CAD build for the part. Positions are in the model's coordinates, mm. A direction names the side the tool comes from. Round coordinates to 2 decimals unless told otherwise and drop trailing zeros. Loops run counter-clockwise (first coordinate to the right, second up) from the corner with the lowest first, then second, coordinate; pieces in that order, holes last.
Autodesk Inventor part; units mm, degrees
ref_plane "Work Plane1" through (0, 9, -50) normal (0, 1, 0) x (-1, 0, 0)
ref_plane "Work Plane2" through (15.25, 0, 0) normal (1, 0, 0) x (0, 1, 0)
ref_plane "YZ Plane" through (0, 0, 0) normal (1, 0, 0) x (0, 1, 0)
sketch "Sketch1" plane through (0, 0, 0) normal (0, 0, 1) x (1, 0, 0)
  circle A0 centre (0, 0) radius 15.25
  dimension "d0" = 30.5
extrude "Extrusion1" add sketch "Sketch1" along normal blind 50
fillet "Fillet1" radius 2 1 edges at (-15.25, 0, 50)
fillet "Fillet2" radius 2 1 edges at (-15.25, 0, 0)
sketch "Sketch2" plane through (0, 0, 50) normal (0, 0, 1) x (1, 0, 0)
  circle A0 centre (0, 0) radius 9
  dimension "d5" = 18
extrude "Extrusion2" add sketch "Sketch2" along normal blind 184
sketch "Sketch3" plane through (0, 0, 0) normal (0, 0, -1) x (-1, 0, 0)
  circle A0 centre (0, 0) radius 9
extrude "Extrusion3" add sketch "Sketch3" along normal blind 50
sketch "Sketch4" plane through (0, 0, -50) normal (0, 0, -1) x (-1, 0, 0)
  circle A0 centre (0, 0) radius 3
  dimension "d10" = 6
extrude "Extrusion4" cut sketch "Sketch4" against normal blind 13
sketch "Sketch5" plane through (0, 0, -50) normal (0, 0, -1) x (-1, 0, 0)
  circle A0 centre (0, 0) radius 9
  point P0 (0, 9)
ref_plane "Work Plane1" through (0, 9, -50) normal (0, 1, 0) x (-1, 0, 0)
sketch "Sketch6" plane through (0, 9, -50) normal (0, 1, 0) x (-1, 0, 0)
  line L0 (-9, 0) -> (9, 0)
  point P0 (0, 50)
  point P1 (0, 5)
  dimension "d13" = 5
hole "Hole1" at (0, 9, -45) direction (0, -1, 0) diameter 3.242 depth 9 tip angle 118
sketch "Sketch7" plane through (0, 0, 0) normal (0, 0, -1) x (-1, 0, 0)
  circle A0 centre (0, 0) radius 15.25
  point P0 (-15.25, 0)
ref_plane "Work Plane2" through (15.25, 0, 0) normal (1, 0, 0) x (0, 1, 0)
sketch "Sketch8" plane through (15.25, 0, 0) normal (1, 0, 0) x (0, 1, 0)
  point P0 (0, 0)
  point P1 (0, 25)
  dimension "d21" = 25
hole "Hole2" at (15.25, 0, 25) direction (-1, 0, 0) diameter 3.242 end through all
sketch "Sketch9" plane through (0, 0, 234) normal (0, 0, 1) x (1, 0, 0)
  circle A0 centre (0, 0) radius 9
  line L0 (2.5, 8.9) -> (2.5, 6.5)
  line L1 (2.5, 6.5) -> (-2.5, 6.5)
  line L2 (-2.5, 6.5) -> (-2.5, 8.6458)
  line L3 (-2.5, 6.5) -> (-2.5, 9)
  line L4 (-2.5, 9) -> (2.5, 9)
  line L5 (2.5, 9) -> (2.5, 6.8873)
  line L6 (-2.5, 9) -> (-2.5, 6.5)
  line L7 (-2.5, 6.5) -> (2.5, 6.5)
  point P0 (0, 6.5)
  point P1 (2.5, 7.7)
  point P2 (2.5, 8.6458)
  dimension "d29" = 5
  dimension "d31" = 0
  dimension "d32" = 2.5
  dimension "d33" = 6.5
  dimension "d34" = 2.5
extrude "Extrusion5" cut sketch "Sketch9" against normal blind 26.5 contours A0 L0 L1 L2 picked at (0, 7.3333)
equation "\"d27\" = Thickness"
equation "\"BendRadius\" = Thickness"
equation "\"BendReliefWidth\" = Thickness"
equation "\"BendReliefDepth\" = 0.5 * Thickness"
equation "\"CornerReliefSize\" = 4 * Thickness"
equation "\"MinimumRemnant\" = 2 * Thickness"
equation "\"TransitionRadius\" = BendRadius"
equation "\"JacobiRadiusSize\" = BendRadius"
equation "\"GapSize\" = Thickness"
properties part number "Final joint shaft"
Item 1: Two-plate mould, pull along Y, no slides. Class faces 1 (the cylindrical face through (-1.172, -8.923, 140.712)), 2 (the flat face through (0, 6.5, 221)), 3 (the flat face through (0, 0, -37)), 4 (the cylindrical face through (0.65, -2.93, -43.59)): released by +Y, released by -Y, zero draft, split by the parting line, or undercut.
Answers follow:
face 1: split by the parting line
face 2: released by +Y
face 3: undercut
face 4: undercut
Item 2: Flat gauge pins, fed straight in: P1, Ø3, axis at x = 0, z = -45, coming from the -Y side; P2, Ø1.7, axis at y = 7, z = 219, coming from the +X side; P3, Ø5, axis at x = -11.5, y = -7.5, coming from the +Z side. Where does each tip first touch, or does it go through?
Answers follow:
P1: stops at y = -9
P2: stops at x = 6.57
P3: stops at z = 50
Item 3: Probe line 1 (Y direction, x = -1, z = 25); line 2 (Z direction, x = 1, y = 0); line 3 (Z direction, x = 4.5, y = -8.5). List the from-to ranges inside material, lowest first.
Answers follow:
line 1: y = -15.22 to -1.62, 1.62 to 15.22
line 2: z = -37 to 23.38, 26.62 to 234
line 3: z = 0 to 50
Item 4: 3-axis set-ups, long thin cutter, end or side, ignore diameter. For faces 5 (the flat face through (9, -3, 50)), 6 (the cylindrical face through (1.172, -8.923, -24.65)), 7 (the flat face through (0, -4, -50)): which of +Z, -Z, +X, -X, +Y, -Y reach the whole face in a straight line?
Answers follow:
face 5: +Z
face 6: -Z
face 7: -Z, +X, -X, +Y, -Y
Item 5: Cut at A-A, the plane z = 167. Give the cut face in (x, y).
Answers follow:
outline: circle Ø18 at (0, 0)
